Verification items for the finished model (mm, model axes). A direction names the side the tool comes from. Give positions to 0.01 mm unless a question says otherwise; leave off trailing zeros. Write each loop counter-clockwise with the first axis right and the second up, starting at its lowest first coordinate (ties: lowest second). Pieces come first, ordered by that corner, then holes. Notation, with made-up numbers: (13, 34.5) - (18, 34.5) arc R6 cw to (18, 38.5) - close; hole circle Ø7 at (47, 61.25). An arc over 180 degrees is marked (long way). Put each result on its own line as item: value.
Autodesk Inventor part; units mm, degrees
ref_plane "YZ Plane" through (0, 0, 0) normal (1, 0, 0) x (0, 1, 0)
ref_plane "XZ Plane" through (0, 0, 0) normal (0, 1, 0) x (-1, 0, 0)
ref_plane "XY Plane" through (0, 0, 0) normal (0, 0, 1) x (1, 0, 0)
sketch "Sketch1" plane through (0, 0, 0) normal (1, 0, 0) x (0, 1, 0)
  line L0 (18.9706, -3.0956) -> (18.9706, 15.9544)
  line L1 (18.9706, 15.9544) -> (23.5426, 15.9544)
  line L2 (23.5426, 15.9544) -> (23.5426, 9.6044)
  line L3 (23.5426, 9.6044) -> (28.3686, 9.6044)
  line L4 (28.3686, 9.6044) -> (28.3686, 8.3344)
  line L5 (28.3686, 8.3344) -> (25.3206, 8.3344)
  line L6 (25.3206, 8.3344) -> (25.3206, -1.8256)
  line L7 (25.3206, -1.8256) -> (28.3686, -1.8256)
  line L8 (28.3686, -1.8256) -> (28.3686, -3.0956)
  line L9 (28.3686, -3.0956) -> (18.9706, -3.0956)
  point P0 (0, 0)
  dimension "d0" = 1.27
  dimension "d1" = 1.27
  dimension "d2" = 10.16
  dimension "d3" = 6.35
  dimension "d6" = 9.398
  dimension "d11" = 6.35
  dimension "d12" = 4.572
revolve "Revolution1" add sketch "Sketch1" angle 360 about axis through (0, 18.9706, -3.0956) along (0, 0, 1)
sketch "Sketch2" plane through (0, 18.9706, -3.0956) normal (0, 0, -1) x (-1, 0, 0)
  circle A0 centre (0, 0) radius 9.398
  circle A1 centre (0, 0) radius 3.3909
  point P0 (0, -18.9706)
  dimension "d8" = 6.7818
extrude "Extrusion1" cut sketch "Sketch2" against normal blind 50.8 contours A1
properties part number "IdlePully"
Q1. Section check D-D, the plane x = 7.5. Record the cut outline in (y, z), plus the area to 3 significant figures.
Answers follow:
outline: (13.31, -3.1) - (24.63, -3.1) - (24.63, -1.83) - (13.31, -1.83) - close; (13.31, 8.33) - (24.63, 8.33) - (24.63, 9.6) - (13.31, 9.6) - close
area: 28.8 mm2
Q2. Set-up check for faces 4 (the face through (-1.751, 23.194, 12.735)), 5 (the face through (6.13, 16.75, 8.334)), 6 (the face through (2, 16, 15.954)): record each of +Z, -Z, +X, -X, +Y, -Y from which the full face is reachable in a straight line by a thin tool's end or side.
Answers follow:
face 4: +Z
face 5: none
face 6: +Z, +X, -X, +Y, -Y
Q3. Section check A-A, the plane x = 0. Record the cut outline in (y, z).
Answers follow:
outline: (9.57, -3.1) - (15.58, -3.1) - (15.58, 15.95) - (14.4, 15.95) - (14.4, 9.6) - (9.57, 9.6) - (9.57, 8.33) - (12.62, 8.33) - (12.62, -1.83) - (9.57, -1.83) - close; (22.36, -3.1) - (28.37, -3.1) - (28.37, -1.83) - (25.32, -1.83) - (25.32, 8.33) - (28.37, 8.33) - (28.37, 9.6) - (23.54, 9.6) - (23.54, 15.95) - (22.36, 15.95) - close
Q4. Section check B-B, the plane y = 11.75. Record the cut outline in (x, z), plus the area to 3 significant figures.
Answers follow:
outline: (-6.02, -3.1) - (6.02, -3.1) - (6.02, -1.83) - (-6.02, -1.83) - close; (-6.02, 8.33) - (6.02, 8.33) - (6.02, 9.6) - (-6.02, 9.6) - close
area: 30.6 mm2
Q5. Go/stop test with flat-tipped pins: pin 1 Ø1.5 at (x, z) = (-4, -1) entering from +Y; pin 2 Ø1 at (x, z) = (-1.5, 0.5) entering from -Y; pin 3 Ø10 at (y, z) = (24.5, 12) entering from -X. Record where each tip stops, or that it passes through.
Answers follow:
pin 1: stops at y = 24.43
pin 2: stops at y = 12.7
pin 3: stops at x = -9.33
Q6. Scan lines: line 1 along Z through (x, y) = (-7, 24.75); line 2 along Y through (x, z) = (0, 4.5); line 3 along X through (y, z) = (18.75, 11). Record each from-to range of solid material in increasing order.
Answers follow:
line 1: z = -3.1 to -1.83, 8.33 to 9.6
line 2: y = 12.62 to 15.58, 22.36 to 25.32
line 3: x = -4.57 to -3.38, 3.38 to 4.57
Q7. Release check for a two-part mould opening along Z. For faces 1 (the face through (0, 23, -3.096)), 2 (the face through (6.13, 16.75, -1.826)), 3 (the face through (0.441, 22.333, 6.296)) record: released by +Z, released by -Z, zero draft, split by the parting line, or undercut.
Answers follow:
face 1: released by -Z
face 2: undercut
face 3: zero draft
Q8. Section check C-C, the plane y = 19.25. Record the cut outline in (x, z), plus the area to 3 significant figures.
Answers follow:
outline: (-9.39, -3.1) - (-3.38, -3.1) - (-3.38, 15.95) - (-4.56, 15.95) - (-4.56, 9.6) - (-9.39, 9.6) - (-9.39, 8.33) - (-6.34, 8.33) - (-6.34, -1.83) - (-9.39, -1.83) - close; (3.38, -3.1) - (9.39, -3.1) - (9.39, -1.83) - (6.34, -1.83) - (6.34, 8.33) - (9.39, 8.33) - (9.39, 9.6) - (4.56, 9.6) - (4.56, 15.95) - (3.38, 15.95) - close
area: 106 mm2
